Can you work these out from the model? Positions are in its coordinate system, mm. A direction names the side the tool comes from. Round coordinates to 2 decimals unless told otherwise and drop trailing zeros. Order: outer loops, then holes, each group sorted by start corner. A loop starts at its lowest first (then second) coordinate and runs counter-clockwise, first axis right, second up.
Q1. We'd pull the mould along X, two halves only. Please class faces 1 (the face through (-1, -4.762, -1)), 2 (the face through (-57.77, -3.91, 70.77)), 3 (the face through (63.5, -4, -10)): pulls with the +X half, pulls with the -X half, needs draft (parallel to the pull), parting line crosses it, or undercut.
Q2. If we section it at C-C (z = 62.5): Please give me the cut outline in (x, y), plus the area to 3 significant figures.
Q3. If we section it at A-A (x = -37.5): Please give me the cut outline in (y, z) (1 decimal).
Q4. If I drill on line 1 (Y direction, x = -54, z = -15); line 2 (Z direction, x = -23, y = -9); line 3 (Z direction, x = -28.5, y = -5) (3 decimals), over which ranges is the centre line in solid material (lowest first)?
Q5. Will these pins go through, and if not, where does the flat tip stop? P1, Ø2.5, axis at x = -4, y = -6.5, coming from the -Z side (3 decimals); P2, Ø11.5, axis at x = -39, z = 19.5, coming from the -Y side.
Q6. If we section it at D-D (x = 49.5): Please give me the cut outline in (y, z).
Q7. If we section it at B-B (z = 10): Please give me the cut outline in (x, y) (1 decimal), plus the area to 3 significant figures.
Q8. For faces 4 (the face through (61, -7.938, 17)), 5 (the face through (-61, -7.938, 17)), 6 (the face through (60.325, -6, -10)), which set-ups out of +Z, -Z, +X, -X, +Y, -Y let a thin tool reach every point of the face, with its end or its side?
from build123d import *

# Parameters (mm, degrees)
F1_DEPTH = 4.7625
F3_DEPTH = 7.9375
F4_W     = 50.8
F4_H     = 3.175
F5_DEPTH = 15.494
F5_TAPER = 2


with BuildPart() as f1:
    # F0 (on Front) → F1 (new body)
    with BuildSketch(Plane.XZ):
        with BuildLine():
            Line((-63.5, -76.2), (63.5, -76.2))
            Line((63.5, -76.2), (63.5, 57.15))
            ThreePointArc((63.5, 57.15), (57.9203841816, 70.6203841816), (44.45, 76.2))
            Line((44.45, 76.2), (-44.45, 76.2))
            ThreePointArc((-44.45, 76.2), (-57.9203841816, 70.6203841816), (-63.5, 57.15))
            Line((-63.5, 57.15), (-63.5, -76.2))
        make_face()
    extrude(amount=F1_DEPTH)

    # F2 (on face) → F3 (join)
    with BuildSketch(Plane(origin=(0, 0, 0), x_dir=(-1, 0, 0), z_dir=(0, 1, 0))):
        with BuildLine():
            ThreePointArc((-44.45, 76.2), (-57.9203841816, 70.6203841816), (-63.5, 57.15))
            Line((-63.5, 57.15), (-63.5, -76.2))
            Line((-63.5, -76.2), (-60.325, -76.2))
            Line((-60.325, -76.2), (-60.325, 57.15))
            ThreePointArc((-60.325, 57.15), (-55.6753201513, 68.3753201513), (-44.45, 73.025))
            Line((-44.45, 73.025), (44.45, 73.025))
            ThreePointArc((44.45, 73.025), (55.6753201513, 68.3753201513), (60.325, 57.15))
            Line((60.325, 57.15), (60.325, -76.2))
            Line((60.325, -76.2), (63.5, -76.2))
            Line((63.5, -76.2), (63.5, 57.15))
            ThreePointArc((63.5, 57.15), (57.9203841816, 70.6203841816), (44.45, 76.2))
            Line((44.45, 76.2), (-44.45, 76.2))
        make_face()
    extrude(amount=-F3_DEPTH)

    # F4 (on face) → F5 (join)
    with BuildSketch(Plane.XZ.offset(7.9375)):
        with Locations((0, 74.6125)):
            Rectangle(F4_W, F4_H)
    extrude(amount=F5_DEPTH, taper=F5_TAPER)


solid = f1.part
Solution:
1. face 1: undercut
1. face 2: pulls with the -X half
1. face 3: pulls with the +X half
2. outline: (-62.73, -7.94) - (-59.4, -7.94) - (-59.4, -4.76) - (59.4, -4.76) - (59.4, -7.94) - (62.73, -7.94) - (62.73, 0) - (-62.73, 0) - close
2. area: 619 mm2
3. outline: (-7.9, 73) - (-4.8, 73) - (-4.8, -76.2) - (0, -76.2) - (0, 76.2) - (-7.9, 76.2) - close
4. line 1: y = -4.76 to 0
4. line 2: z = 73.06 to 76.16
4. line 3: z = 73.025 to 76.2
5. P1: stops at z = 73.025
5. P2: stops at y = -4.76
6. outline: (-7.94, 72.2) - (-4.76, 72.2) - (-4.76, -76.2) - (0, -76.2) - (0, 75.52) - (-7.94, 75.52) - close
7. outline: (-63.5, -7.9) - (-60.3, -7.9) - (-60.3, -4.8) - (60.3, -4.8) - (60.3, -7.9) - (63.5, -7.9) - (63.5, 0) - (-63.5, 0) - close
7. area: 625 mm2
8. face 4: +Z, -Z, +X, -Y
8. face 5: +Z, -Z, -X, -Y
8. face 6: -Z, -Y
